Autodesk Inventor part; units mm, degrees
ref_plane "YZ Plane" through (0, 0, 0) normal (1, 0, 0) x (0, 1, 0)
ref_plane "XZ Plane" through (0, 0, 0) normal (0, 1, 0) x (-1, 0, 0)
ref_plane "XY Plane" through (0, 0, 0) normal (0, 0, 1) x (1, 0, 0)
sketch "Sketch1" plane through (0, 0, 0) normal (0, 1, 0) x (-1, 0, 0)
  line L0 (12.7, 76.2) -> (-12.7, 76.2)
  line L1 (-12.7, 76.2) -> (-12.7, -76.2)
  line L2 (-12.7, -76.2) -> (12.7, -76.2)
  line L3 (12.7, -76.2) -> (12.7, 76.2)
  line L4 (12.7, 76.2) -> (-12.7, -76.2) construction
  line L5 (-12.7, 76.2) -> (12.7, -76.2) construction
  point P0 (0, 0)
  dimension "d0" = 25.4
  dimension "d1" = 152.4
extrude "Extrusion1" add sketch "Sketch1" along normal blind 12.7
sketch "Sketch2" plane through (-12.7, 0, 76.2) normal (0, 0, 1) x (1, 0, 0)
  line L0 (0, 0) -> (25.4, 0)
  line L1 (25.4, 0) -> (25.4, 12.7)
  line L2 (0, 12.7) -> (25.4, 12.7)
  line L3 (0, 0) -> (0, 12.7)
  line L4 (3.175, 12.7) -> (22.225, 12.7)
  line L5 (22.225, 12.7) -> (22.225, 6.35)
  line L6 (22.225, 6.35) -> (3.175, 6.35)
  line L7 (3.175, 6.35) -> (3.175, 12.7)
  point P0 (12.7, 0)
  dimension "d4" = 3.175
  dimension "d5" = 6.35
  dimension "d6" = 3.175
extrude "Extrusion2" cut sketch "Sketch2" against normal through all contours L2 L5 L6 L7
equation "\"d6\" = d4"
properties part number "Base"
Work out the finished part from the listing and answer in its coordinate system (mm). A direction names the side the tool comes from. Give positions to 0.01 mm unless a question says otherwise; leave off trailing zeros. Write each loop counter-clockwise with the first axis right and the second up, starting at its lowest first coordinate (ties: lowest second). Pieces come first, ordered by that corner, then holes. Notation, with made-up numbers: (61.25, 25) - (113.25, 25) arc R14 cw to (113.25, 39) - close; hole circle Ø1 at (24.25, -24). An arc over 180 degrees is marked (long way). One line per item, written item: value. Start each with the question number.
1. Find section A-A (y = 10.5). Write down the section's boundary in (x, z) (3 decimals).
2. Consider probe 1 along X at (y, z) = (6.5, 30) (3 decimals); probe 2 along Y at (x, z) = (-1.5, 1.5). Determine where each line is inside the solid, lowest interval first.
3. Given pin 1 (9.5 mm diameter, centred on x = 2, z = -22, fed in from +Y), flat-ended and moving along its own axis, determine where the tip first touches the part or whether it passes through.
4. Find section B-B (z = -12). Write down the section's boundary in (x, y) (3 decimals), then the cut area to 3 significant figures.
5. Find section C-C (x = -3). Write down the section's boundary in (y, z), then the cut area to 3 significant figures.
6. For faces 1 (the flat face through (0, 0, 1)), 2 (the flat face through (9.525, 10, 1)), determine the directions among +Z, -Z, +X, -X, +Y, -Y from which every point of the face is accessible in a straight line to the end or side of a thin tool.
Geometry results:
1. outline: (-12.7, -76.2) - (-9.525, -76.2) - (-9.525, 76.2) - (-12.7, 76.2) - close; (9.525, -76.2) - (12.7, -76.2) - (12.7, 76.2) - (9.525, 76.2) - close
2. probe 1: -12.7 to -9.525, 9.525 to 12.7
2. probe 2: 0 to 6.35
3. pin 1: y = 6.35
4. outline: (-12.7, 0) - (12.7, 0) - (12.7, 12.7) - (9.525, 12.7) - (9.525, 6.35) - (-9.525, 6.35) - (-9.525, 12.7) - (-12.7, 12.7) - close
4. area: 202 mm2
5. outline: (0, -76.2) - (6.35, -76.2) - (6.35, 76.2) - (0, 76.2) - close
5. area: 968 mm2
6. face 1: +Z, -Z, +X, -X, -Y
6. face 2: +Z, -Z, +Y
